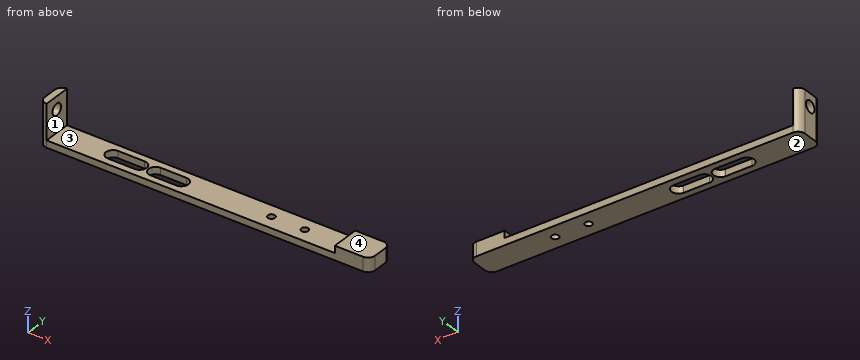
Autodesk Fusion 360 part; units mm, degrees
sketch "Sketch1" plane through (0, 0, 0) normal (0, 0, 1) x (1, 0, 0)
  line L0 (-70, 20) -> (165, 20)
  line L1 (165, 20) -> (165, 0)
  line L2 (165, 0) -> (-70, 0)
  line L3 (-70, 0) -> (-70, 20)
  dimension "d1" = 235
  dimension "d2" = 20
extrude "Extrude1" add sketch "Sketch1" along normal blind 5
sketch "Sketch2" plane through (0, 0, 5) normal (0, 0, 1) x (-1, 0, 0)
  line L0 (70, 0) -> (-165, 0)
  line L1 (-165, 0) -> (-165, -20)
  line L2 (-165, -20) -> (70, -20)
  line L3 (70, -20) -> (70, 0)
  circle A0 centre (-87.5581, -10.1163) radius 2.5
  circle A1 centre (-111.2788, -10.1163) radius 2.5
  line L4 (25.0313, -5.0352) -> (6.1177, -5.0352)
  arc A2 (6.1177, -5.0352) -> (6.1177, -15.0352) centre (6.1177, -10.0352) ccw
  line L5 (6.1177, -15.0352) -> (25.0313, -15.0352)
  arc A3 (25.0313, -15.0352) -> (25.0313, -5.0352) centre (25.0313, -10.0352) ccw
  line L6 (25.0313, -10.0352) -> (6.1177, -10.0352) construction
  line L7 (-5.3429, -4.8835) -> (-23.6696, -4.8835)
  arc A4 (-23.6696, -4.8835) -> (-23.6696, -14.8835) centre (-23.6696, -9.8835) ccw
  line L8 (-23.6696, -14.8835) -> (-5.3429, -14.8835)
  arc A5 (-5.3429, -14.8835) -> (-5.3429, -4.8835) centre (-5.3429, -9.8835) ccw
  line L9 (-5.3429, -9.8835) -> (-23.6696, -9.8835) construction
  point P0 (6.1177, -10.0352)
  dimension "d5" = 5
  dimension "d6" = 5
  dimension "d7" = 10
  dimension "d8" = 10
extrude "Extrude2" cut sketch "Sketch2" against normal blind 20 contours A0 | A1 | L4 A2 L5 A3 | L7 A4 L8 A5
fillet "Fillet1" radius 5 4 edges at (165, 0, 2.5) (165, 20, 2.5) (-70, 20, 2.5) (-70, 0, 2.5)
sketch "Sketch3" plane through (0, 0, 5) normal (0, 0, 1) x (-1, 0, 0)
  arc A0 (70, -5) -> (65, 0) centre (65, -5) ccw
  line L0 (65, 0) -> (-160, 0)
  arc A1 (-160, 0) -> (-165, -5) centre (-160, -5) ccw
  line L1 (-165, -5) -> (-165, -15)
  arc A2 (-165, -15) -> (-160, -20) centre (-160, -15) ccw
  line L2 (-160, -20) -> (65, -20)
  arc A3 (65, -20) -> (70, -15) centre (65, -15) ccw
  line L3 (70, -15) -> (70, -5)
  line L4 (6.1177, -5.0352) -> (25.0313, -5.0352)
  arc A4 (25.0313, -15.0352) -> (25.0313, -5.0352) centre (25.0313, -10.0352) ccw
  line L5 (25.0313, -15.0352) -> (6.1177, -15.0352)
  arc A5 (6.1177, -5.0352) -> (6.1177, -15.0352) centre (6.1177, -10.0352) ccw
  circle A6 centre (-111.2788, -10.1163) radius 2.5
  line L6 (-23.6696, -4.8835) -> (-5.3429, -4.8835)
  arc A7 (-5.3429, -14.8835) -> (-5.3429, -4.8835) centre (-5.3429, -9.8835) ccw
  line L7 (-5.3429, -14.8835) -> (-23.6696, -14.8835)
  arc A8 (-23.6696, -4.8835) -> (-23.6696, -14.8835) centre (-23.6696, -9.8835) ccw
  circle A9 centre (-87.5581, -10.1163) radius 2.5
  line L8 (-165, -20) -> (-140, -20)
  line L9 (-140, -20) -> (-140, 0)
  line L10 (-140, 0) -> (-165, 0)
  line L11 (-165, 0) -> (-165, -20)
  dimension "d13" = 25
  dimension "d14" = 20
extrude "Extrude3" add sketch "Sketch3" along normal blind 5 contours L0 A1 L1 A2 L2 L8 L9 L10 L11
sketch "Sketch4" plane through (0, 0, 5) normal (0, 0, 1) x (-1, 0, 0)
  line L0 (-140, 0) -> (-140, -20)
  line L1 (-140, -20) -> (65, -20)
  arc A0 (65, -20) -> (70, -15) centre (65, -15) ccw
  line L2 (70, -15) -> (70, -5)
  arc A1 (70, -5) -> (65, 0) centre (65, -5) ccw
  line L3 (65, 0) -> (-140, 0)
  line L4 (6.1177, -5.0352) -> (25.0313, -5.0352)
  arc A2 (25.0313, -15.0352) -> (25.0313, -5.0352) centre (25.0313, -10.0352) ccw
  line L5 (25.0313, -15.0352) -> (6.1177, -15.0352)
  arc A3 (6.1177, -5.0352) -> (6.1177, -15.0352) centre (6.1177, -10.0352) ccw
  circle A4 centre (-111.2788, -10.1163) radius 2.5
  line L6 (-23.6696, -4.8835) -> (-5.3429, -4.8835)
  arc A5 (-5.3429, -14.8835) -> (-5.3429, -4.8835) centre (-5.3429, -9.8835) ccw
  line L7 (-5.3429, -14.8835) -> (-23.6696, -14.8835)
  arc A6 (-23.6696, -4.8835) -> (-23.6696, -14.8835) centre (-23.6696, -9.8835) ccw
  circle A7 centre (-87.5581, -10.1163) radius 2.5
  line L8 (70, -20) -> (65, -20)
  line L9 (65, -20) -> (65, 0)
  line L10 (65, 0) -> (70, 0)
  line L11 (70, 0) -> (70, -20)
  dimension "d17" = 5
  dimension "d18" = 20
extrude "Extrude4" add sketch "Sketch4" along normal blind 25 contours A0 L2 A1 L9 L11
sketch "Sketch5" plane through (-65, 0, 0) normal (1, 0, 0) x (0, 1, 0)
  line L0 (0, 5) -> (20, 5)
  line L1 (20, 5) -> (20, 30)
  line L2 (20, 30) -> (0, 30)
  line L3 (0, 30) -> (0, 5)
  circle A0 centre (10, 21) radius 4.15
  dimension "d21" = 8.3
  dimension "d22" = 16
extrude "Extrude5" cut sketch "Sketch5" against normal blind 6 contours A0
thread "Thread1" thread offset 0 thread length 10
thread "Thread2" thread offset 0 thread length 10
Could you check a few things on this model? Use its own coordinates, in mm. Face numbers are marked on the shaded views. A direction names the side the tool comes from. Give positions to 0.01 mm unless a question says otherwise; leave off trailing zeros. Order: outer loops, then holes, each group sorted by start corner. A loop starts at its lowest first (then second) coordinate and runs counter-clockwise, first axis right, second up. Notation, with made-up numbers: (6, 28) -> (12, 28) arc R22 ccw to (12, 56) -> close; hole circle Ø7 at (-10.75, 72.25). An arc over 180 degrees is marked (long way). Answer in a Markdown table with one row per item. Add a question column.
Item 1: Please list where these lines run through material, in increasing order: probe 1 along X at (y, z) = (10.5, 7); probe 2 along Z at (x, y) = (107.5, 8.5); probe 3 along X at (y, z) = (8, 2).
Item 2: I'm going to push flat-ended pins straight in: P1, Ø12, axis at x = 59, y = 17, coming from the +Z side; P2, Ø1, axis at y = 3, z = 26, coming from the -X side; P3, Ø12, axis at y = 13.5, z = 26.5, coming from the +X side; P4, Ø5.5, axis at x = 17, z = 2, coming from the -Y side. Where does each tip first touch, or does it pass through?
Item 3: Imagine slicing it at B-B (z = 21). List the corners of the cut face in (x, y) for me.
Item 4: Imagine slicing it at C-C (x = 47). List the corners of the cut face in (y, z) for me, and give its area (3 significant figures).
Item 5: For the marked faces 3 and 4, which set-ups out of +Z, -Z, +X, -X, +Y, -Y let a thin tool reach every point of the face, with its end or its side?
Item 6: Imagine slicing it at A-A (z = 7.5). List the corners of the cut face in (x, y) for me.
Item 7: We'd pull the mould along X, two halves only. Please class the marked faces 1 and 2: pulls with the +X half, pulls with the -X half, needs draft (parallel to the pull), parting line crosses it, or undercut.
Item 8: Imagine slicing it at D-D (y = 17.5). List the corners of the cut face in (x, z) for me, and give its area (3 significant figures).
Result:
| question | item | result |
|---|---|---|
| 1 | probe 1 | -70 to -65, 140 to 165 |
| 1 | probe 2 | 0 to 5 |
| 1 | probe 3 | -70 to -29.6, -1.55 to 0.71, 28.3 to 86.23, 88.89 to 109.95, 112.61 to 165 |
| 2 | P1 | z = 5 |
| 2 | P2 | x = -69.77 |
| 2 | P3 | x = -65 |
| 2 | P4 | y = 0 |
| 3 | outline | (-70, 5) arc R5 ccw to (-65, 0) -> (-65, 5.85) -> (-70, 5.85) -> close; (-70, 14.15) -> (-65, 14.15) -> (-65, 20) arc R5 ccw to (-70, 15) -> close |
| 4 | outline | (0, 0) -> (20, 0) -> (20, 5) -> (0, 5) -> close |
| 4 | area | 100 mm2 |
| 5 | face 3 | +Z, +Y, -Y |
| 5 | face 4 | +Z, +X, +Y, -Y |
| 6 | outline | (-70, 5) arc R5 ccw to (-65, 0) -> (-65, 20) arc R5 ccw to (-70, 15) -> close; (140, 0) -> (160, 0) arc R5 ccw to (165, 5) -> (165, 15) arc R5 ccw to (160, 20) -> (140, 20) -> close |
| 7 | face 1 | undercut |
| 7 | face 2 | needs draft |
| 8 | outline | (-69.33, 0) -> (164.33, 0) -> (164.33, 10) -> (140, 10) -> (140, 5) -> (-65, 5) -> (-65, 30) -> (-69.33, 30) -> close |
| 8 | area | 1,400 mm2 |
